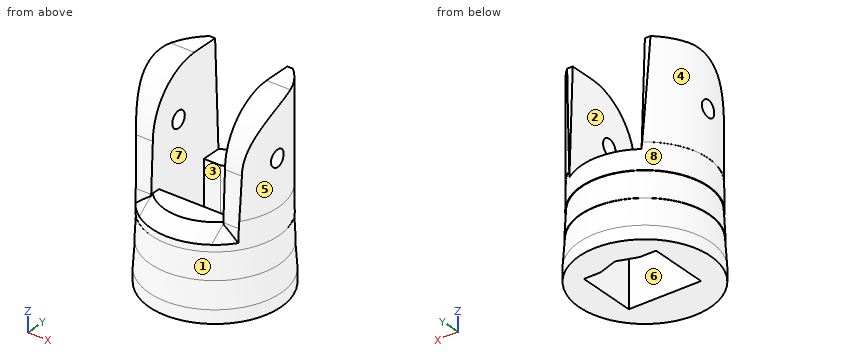
```python
from build123d import *

# Parameters (mm, degrees)
SKETCH2_R               = 10
BOSS_EXTRUDE1_DEPTH     = 2
SKETCH3_R               = 10
BOSS_EXTRUDE2_DEPTH     = 4
BOSS_EXTRUDE2_TAPER     = 4
SKETCH4_R               = 9.790219564
BOSS_EXTRUDE3_DEPTH     = 4
BOSS_EXTRUDE3_TAPER     = 3
SKETCH5_R               = 9.685404006
BOSS_EXTRUDE4_DEPTH     = 4
BOSS_EXTRUDE4_TAPER     = 1
SKETCH6_R               = 9.633038811
BOSS_EXTRUDE5_DEPTH     = 15
CUT_EXTRUDE1_DEPTH      = 14
CUT_EXTRUDE1_DEPTH_BACK = 14
SKETCH7_W               = 11
SKETCH7_H               = 17.89942169
CUT_EXTRUDE4_DEPTH      = 14
CUT_EXTRUDE5_DEPTH      = 10
CUT_EXTRUDE5_DEPTH_BACK = 10
CHAMFER1_SIZE           = 2
CUT_EXTRUDE6_DEPTH      = 10
CUT_EXTRUDE6_DEPTH_BACK = 10
SKETCH11_R              = 1.25


with BuildPart() as part:
    # Sketch2 → Boss-Extrude1 (new body)
    with BuildSketch(Plane.XY):
        Circle(SKETCH2_R)
    extrude(amount=BOSS_EXTRUDE1_DEPTH)

    # Sketch3 → Boss-Extrude2 (add)
    with BuildSketch(Plane.XY.offset(2)):
        Circle(SKETCH3_R)
    extrude(amount=BOSS_EXTRUDE2_DEPTH, taper=BOSS_EXTRUDE2_TAPER)

    # Sketch4 → Boss-Extrude3 (add)
    with BuildSketch(Plane.XY.offset(6)):
        Circle(SKETCH4_R)
    extrude(amount=BOSS_EXTRUDE3_DEPTH, taper=BOSS_EXTRUDE3_TAPER)

    # Sketch5 → Boss-Extrude4 (add)
    with BuildSketch(Plane.XY.offset(10)):
        Circle(SKETCH5_R)
    extrude(amount=BOSS_EXTRUDE4_DEPTH, taper=BOSS_EXTRUDE4_TAPER)

    # Sketch6 → Boss-Extrude5 (add)
    with BuildSketch(Plane.XY.offset(14)):
        Circle(SKETCH6_R)
    extrude(amount=BOSS_EXTRUDE5_DEPTH)

    # Sketch7 → Cut-Extrude1 (cut, two sides: drawn at the far end of the back side and taken through both)
    with BuildSketch(Plane(origin=(0, 0, 0), x_dir=(1, 0, 0), z_dir=(0, 1, 0)).offset(-CUT_EXTRUDE1_DEPTH_BACK)):
        with Locations((0, -21.949710845)):
            Rectangle(SKETCH7_W, SKETCH7_H)
    extrude(amount=CUT_EXTRUDE1_DEPTH + CUT_EXTRUDE1_DEPTH_BACK, mode=Mode.SUBTRACT)

    # Sketch10 → Cut-Extrude4 (cut)
    with BuildSketch(Plane(origin=(0, 0, 0), x_dir=(-1, 0, 0), z_dir=(0, 0, -1))):
        Polygon((-5.5, 5), (-5.5, -4), (5.5, -4), (5.5, 5), (3, 5), (0, 6), (-3, 5), align=None)
    extrude(amount=-CUT_EXTRUDE4_DEPTH, mode=Mode.SUBTRACT)

    # Sketch8 → Cut-Extrude5 (cut, two sides: drawn at the far end of the back side and taken through both)
    with BuildSketch(Plane(origin=(0, 0, 0), x_dir=(0, 0, -1), z_dir=(1, 0, 0)).offset(-CUT_EXTRUDE5_DEPTH_BACK)):
        with BuildLine():
            Line((-13, 9.633038811), (-13, 7.9085673))
            Line((-13, 7.9085673), (-29, 7.240766023))
            Line((-29, 7.240766023), (-29, 3.070766023))
            ThreePointArc((-29, 3.070766023), (-26.359814718, -2.832037351), (-20.36, -5.243652859))
            Line((-20.36, -5.243652859), (-13, -5.5714327))
            Line((-13, -5.5714327), (-13, -9.633038811))
            Line((-13, -9.633038811), (-33.781866843, -9.633038811))
            Line((-33.781866843, -9.633038811), (-33.781866843, 9.633038811))
            Line((-33.781866843, 9.633038811), (-13, 9.633038811))
        make_face()
    extrude(amount=CUT_EXTRUDE5_DEPTH + CUT_EXTRUDE5_DEPTH_BACK, mode=Mode.SUBTRACT)

    # Chamfer1
    # the kernel refuses this chamfer: 2 mm, written as the material it takes off along each edge
    with BuildSketch(Plane(origin=(0, 0, 13), x_dir=(0.9966107214684086, -0.08226220185612716, 1.2908177907304536e-15), z_dir=(0.08226220185612716, 0.9966107214684086, 1.0371882149808466e-15))) as chamfer1_piece_1_section:
        Polygon((9.633038811 + CHAMFER1_SIZE * 0.0174524064373, CHAMFER1_SIZE * 0.999847695156), (9.633038811 - CHAMFER1_SIZE, 0), (9.633038811, 0), align=None)
    chamfer1_piece_1 = revolve(axis=Axis((0, 0, 13), (0, 0, -1)), revolution_arc=170.562781842, mode=Mode.PRIVATE)
    chamfer1_piece_1 = split(chamfer1_piece_1, bisect_by=Plane(origin=(-5.5, -5.504615156, 12.950413225), z_dir=(1, 0, 0)), keep=Keep.TOP, mode=Mode.PRIVATE)
    chamfer1_piece_1 = split(chamfer1_piece_1, bisect_by=Plane(origin=(5.5, -5.504615156, 12.950413225), z_dir=(-1, 0, 0)), keep=Keep.TOP, mode=Mode.PRIVATE)
    add(chamfer1_piece_1, mode=Mode.SUBTRACT)
    with BuildSketch(Plane(origin=(0, 0, 13), x_dir=(0.9966107214684086, -0.08226220185612716, 1.2908177907304536e-15), z_dir=(0.08226220185612716, 0.9966107214684086, 1.0371882149808466e-15))) as chamfer1_piece_2_section:
        Polygon((9.633038811 + CHAMFER1_SIZE * 0.0174524064373, CHAMFER1_SIZE * 0.999847695156), (9.633038811 - CHAMFER1_SIZE, 0), (9.633038811, 0), align=None)
    chamfer1_piece_2 = revolve(axis=Axis((0, 0, 13), (0, 0, -1)), revolution_arc=170.562781842, mode=Mode.PRIVATE)
    chamfer1_piece_2 = split(chamfer1_piece_2, bisect_by=Plane(origin=(6.416338432, -5.607046409, 12.200326364), z_dir=(0, -0.9990097760809877, 0.04449120468828483)), keep=Keep.TOP, mode=Mode.PRIVATE)
    add(chamfer1_piece_2, mode=Mode.SUBTRACT)

    # Sketch11 → Cut-Extrude6 (cut, two sides: drawn at the far end of the back side and taken through both)
    with BuildSketch(Plane(origin=(0, 0, 0), x_dir=(0, 0, -1), z_dir=(1, 0, 0)).offset(-CUT_EXTRUDE6_DEPTH_BACK)):
        with Locations(Location((-21, -0.0914327, 0), (0, 0, 180))):
            Circle(SKETCH11_R)
    extrude(amount=CUT_EXTRUDE6_DEPTH + CUT_EXTRUDE6_DEPTH_BACK, mode=Mode.SUBTRACT)


solid = part.part
```
Work out the finished part from the listing and answer in its coordinate system (mm). Face numbers are marked on the shaded views. A direction names the side the tool comes from. Round coordinates to 2 decimals unless told otherwise and drop trailing zeros. Write each loop counter-clockwise with the first axis right and the second up, starting at its lowest first coordinate (ties: lowest second). Pieces come first, ordered by that corner, then holes.
1) Determine the mould class of the marked faces 5, 6, 7 and 8 for opening direction X: pulls with the +X half, pulls with the -X half, needs draft (parallel to the pull), parting line crosses it, or undercut.
2) Which of the six approach directions +Z, -Z, +X, -X, +Y, -Y give full straight-line access (tool end or side, diameter ignored) to the marked faces 1, 2, 3 and 4?
3) Consider probe 1 along X at (y, z) = (7, 17.75); probe 2 along Y at (x, z) = (0.5, 4); probe 3 along X at (y, z) = (2, 7.75). Determine where each line is inside the solid, lowest interval first.
4) A cutting plane is placed at A-A on z = 21. Determine the outline of the cut face in (x, y), and give its area (3 significant figures).
5) Flat-ended cylindrical pins translate along their axes: P1, Ø3, axis at y = 4.5, z = 22, coming from the +X side; P2, Ø0.8, axis at x = -4.5, z = 4, coming from the -Y side; P3, Ø3.5, axis at x = 2.5, y = 7.5, coming from the +Z side; P4, Ø2, axis at y = -0.09, z = 21, coming from the -X side. Find the tip coordinate at first contact, or state that the pin passes through.
6) A cutting plane is placed at B-B on z = 24.5. Determine the outline of the cut face in (x, y).
Entries:
1. face 5: pulls with the +X half
1. face 6: undercut
1. face 7: undercut
1. face 8: parting line crosses it
2. face 1: none
2. face 2: +Z
2. face 3: +Z, -Z
2. face 4: +Z, -X
3. probe 1: x = -6.62 to -5.5, 5.5 to 6.62
3. probe 2: y = -9.85 to -4, 5.83 to 9.85
3. probe 3: x = -9.49 to -5.5, 5.5 to 9.49
4. outline: (-9.56, 1.16) - (-5.5, 1.16) - (-5.5, 7.57) - (-5.95, 7.57) arc R9.63 ccw to start; (-9.54, -1.34) arc R9.63 ccw to (-8.1, -5.22) - (-5.5, -5.22) - (-5.5, -1.34) - close; (5.5, -5.22) - (8.1, -5.22) arc R9.63 ccw to (9.54, -1.34) - (5.5, -1.34) - close; (5.5, 1.16) - (9.56, 1.16) arc R9.63 ccw to (5.95, 7.57) - (5.5, 7.57) - close
4. area: 63.2 mm2
5. P1: stops at x = 9.15
5. P2: stops at y = -8.97
5. P3: stops at z = 13
5. P4: passes through
6. outline: (-8.67, -4.19) - (-5.5, -4.19) - (-5.5, 7.43) - (-6.13, 7.43) arc R9.63 ccw to start; (5.5, -4.19) - (8.67, -4.19) arc R9.63 ccw to (6.13, 7.43) - (5.5, 7.43) - close
